from build123d import *

# Parameters (mm, degrees)
BOSS_EXTRUDE1_DEPTH = 6
BOSS_EXTRUDE2_DEPTH = 2.5
BOSS_EXTRUDE4_DEPTH = 2.5
BOSS_EXTRUDE5_DEPTH = 2.5
FILLET1_R           = 2.5
SKETCH6_R           = 2.2
CUT_EXTRUDE1_DEPTH  = 105.505992651
CHAMFER1_SIZE       = 2
SKETCH8_R           = 1.25
BOSS_EXTRUDE6_DEPTH = 2.5
SKETCH10_W          = 2.5
SKETCH10_H          = 5
BOSS_EXTRUDE8_DEPTH = 7.5
SKETCH11_W          = 5
SKETCH11_H          = 2.5
BOSS_EXTRUDE9_DEPTH = 15
FILLET2_R           = 1


with BuildPart() as part:
    # Sketch1 → Boss-Extrude1 (new body)
    with BuildSketch(Plane(origin=(0, 0, 0), x_dir=(1, 0, 0), z_dir=(0, 1, 0))):
        with BuildLine():
            Line((44.658133395, 16.413194813), (15.158133395, 28.913194813))
            ThreePointArc((15.158133395, 28.913194813), (14.345997058, 29.164947656), (13.5, 29.25))
            Line((13.5, 29.25), (-13.5, 29.25))
            ThreePointArc((-13.5, 29.25), (-14.345997058, 29.164947656), (-15.158133395, 28.913194813))
            Line((-15.158133395, 28.913194813), (-44.658133395, 16.413194813))
            ThreePointArc((-44.658133395, 16.413194813), (-46.543272988, 14.846852474), (-47.25, 12.5))
            Line((-47.25, 12.5), (-47.25, -12.5))
            ThreePointArc((-47.25, -12.5), (-46.543272988, -14.846852474), (-44.658133395, -16.413194813))
            Line((-44.658133395, -16.413194813), (-15.158133395, -28.913194813))
            ThreePointArc((-15.158133395, -28.913194813), (-14.345997058, -29.164947656), (-13.5, -29.25))
            Line((-13.5, -29.25), (13.5, -29.25))
            ThreePointArc((13.5, -29.25), (14.345997058, -29.164947656), (15.158133395, -28.913194813))
            Line((15.158133395, -28.913194813), (44.658133395, -16.413194813))
            ThreePointArc((44.658133395, -16.413194813), (46.543272988, -14.846852474), (47.25, -12.5))
            Line((47.25, -12.5), (47.25, 12.5))
            ThreePointArc((47.25, 12.5), (46.543272988, 14.846852474), (44.658133395, 16.413194813))
        make_face()
        with BuildLine():
            Line((43.68276081, 14.111315511), (14.18276081, 26.611315511))
            ThreePointArc((14.18276081, 26.611315511), (13.84835173, 26.714978447), (13.5, 26.75))
            Line((13.5, 26.75), (-13.5, 26.75))
            ThreePointArc((-13.5, 26.75), (-13.84835173, 26.714978447), (-14.18276081, 26.611315511))
            Line((-14.18276081, 26.611315511), (-43.68276081, 14.111315511))
            ThreePointArc((-43.68276081, 14.111315511), (-44.45899476, 13.466351019), (-44.75, 12.5))
            Line((-44.75, 12.5), (-44.75, -12.5))
            ThreePointArc((-44.75, -12.5), (-44.45899476, -13.466351019), (-43.68276081, -14.111315511))
            Line((-43.68276081, -14.111315511), (-14.18276081, -26.611315511))
            ThreePointArc((-14.18276081, -26.611315511), (-13.84835173, -26.714978447), (-13.5, -26.75))
            Line((-13.5, -26.75), (13.5, -26.75))
            ThreePointArc((13.5, -26.75), (13.84835173, -26.714978447), (14.18276081, -26.611315511))
            Line((14.18276081, -26.611315511), (43.68276081, -14.111315511))
            ThreePointArc((43.68276081, -14.111315511), (44.45899476, -13.466351019), (44.75, -12.5))
            Line((44.75, -12.5), (44.75, 12.5))
            ThreePointArc((44.75, 12.5), (44.45899476, 13.466351019), (43.68276081, 14.111315511))
        make_face(mode=Mode.SUBTRACT)
    extrude(amount=BOSS_EXTRUDE1_DEPTH)

    # Sketch2 → Boss-Extrude2 (add)
    with BuildSketch(Plane(origin=(0, 6, 0), x_dir=(1, 0, 0), z_dir=(0, 1, 0))):
        with BuildLine():
            Line((-44.658133395, -16.413194813), (-15.158133395, -28.913194813))
            ThreePointArc((-15.158133395, -28.913194813), (-14.345997058, -29.164947656), (-13.5, -29.25))
            Line((-13.5, -29.25), (13.5, -29.25))
            ThreePointArc((13.5, -29.25), (14.345997058, -29.164947656), (15.158133395, -28.913194813))
            Line((15.158133395, -28.913194813), (44.658133395, -16.413194813))
            ThreePointArc((44.658133395, -16.413194813), (46.543272988, -14.846852474), (47.25, -12.5))
            Line((47.25, -12.5), (47.25, 12.5))
            ThreePointArc((47.25, 12.5), (46.543272988, 14.846852474), (44.658133395, 16.413194813))
            Line((44.658133395, 16.413194813), (15.158133395, 28.913194813))
            ThreePointArc((15.158133395, 28.913194813), (14.345997058, 29.164947656), (13.5, 29.25))
            Line((13.5, 29.25), (-13.5, 29.25))
            ThreePointArc((-13.5, 29.25), (-14.345997058, 29.164947656), (-15.158133395, 28.913194813))
            Line((-15.158133395, 28.913194813), (-44.658133395, 16.413194813))
            ThreePointArc((-44.658133395, 16.413194813), (-46.543272988, 14.846852474), (-47.25, 12.5))
            Line((-47.25, 12.5), (-47.25, -12.5))
            ThreePointArc((-47.25, -12.5), (-46.543272988, -14.846852474), (-44.658133395, -16.413194813))
        make_face()
    extrude(amount=BOSS_EXTRUDE2_DEPTH)

    # Sketch4 → Boss-Extrude4 (add)
    with BuildSketch(Plane(origin=(47.25, 0, 0), x_dir=(0, 0, -1), z_dir=(1, 0, 0))):
        Polygon((-7.5, 0), (7.5, 0), (5, -33.7), (-5, -33.7), align=None)
    extrude(amount=-BOSS_EXTRUDE4_DEPTH)

    # Sketch5 → Boss-Extrude5 (add)
    with BuildSketch(Plane.ZY.offset(47.25)):
        Polygon((7.5, 0), (5, -33.7), (-5, -33.7), (-7.5, 0), align=None)
    extrude(amount=-BOSS_EXTRUDE5_DEPTH)

    # Fillet1
    fillet1_edges = [part.edges().sort_by_distance(p)[0] for p in [
        (46, -33.7, -5),
        (46, 0, -7.5),
        (46, 0, 7.5),
        (46, -33.7, 5),
        (-46, -33.7, -5),
        (-46, -33.7, 5),
        (-46, 0, 7.5),
        (-46, 0, -7.5),
    ]]
    fillet(fillet1_edges, radius=FILLET1_R)

    # Sketch6 → Cut-Extrude1 (cut, through all)
    with BuildSketch(Plane(origin=(47.25, 0, 0), x_dir=(0, 0, -1), z_dir=(1, 0, 0))):
        with Locations((0, -2.3)):
            Circle(SKETCH6_R)
        with Locations((0, -27.7)):
            Circle(SKETCH6_R)
    extrude(amount=-CUT_EXTRUDE1_DEPTH, mode=Mode.SUBTRACT)

    # Chamfer1
    chamfer1_edges = [part.edges().sort_by_distance(p)[0] for p in [
        (-47.25, -2.3, 2.2),
        (47.25, -2.3, 2.2),
        (-47.25, -27.7, 2.2),
        (47.25, -27.7, 2.2),
    ]]
    chamfer(chamfer1_edges, length=CHAMFER1_SIZE)

    # Sketch8 → Boss-Extrude6 (add)
    with BuildSketch(Plane(origin=(0, 6, 0), x_dir=(-1, 0, 0), z_dir=(0, -1, 0))):
        with Locations(Location((40, 10.512979117, 0), (0, 0, 270))):
            Circle(SKETCH8_R)
        with Locations(Location((16.5, 20.470606235, 0), (0, 0, 270))):
            Circle(SKETCH8_R)
        with Locations(Location((-16.5, -20.470606235, 0), (0, 0, 270))):
            Circle(SKETCH8_R)
        with Locations(Location((-40, -10.512979117, 0), (0, 0, 270))):
            Circle(SKETCH8_R)
        with Locations(Location((-40, 10.512979117, 0), (0, 0, 270))):
            Circle(SKETCH8_R)
        with Locations(Location((-16.5, 20.470606235, 0), (0, 0, 270))):
            Circle(SKETCH8_R)
        with Locations(Location((40, -10.512979117, 0), (0, 0, 270))):
            Circle(SKETCH8_R)
        with Locations(Location((16.5, -20.470606235, 0), (0, 0, 270))):
            Circle(SKETCH8_R)
    extrude(amount=BOSS_EXTRUDE6_DEPTH)

    # Sketch10 → Boss-Extrude8 (add)
    with BuildSketch(Plane(origin=(0, 6, 0), x_dir=(-1, 0, 0), z_dir=(0, -1, 0))):
        with Locations((7.5, 0)):
            Rectangle(SKETCH10_W, SKETCH10_H)
    extrude(amount=BOSS_EXTRUDE8_DEPTH)

    # Sketch11 → Boss-Extrude9 (add)
    with BuildSketch(Plane.ZY.offset(6.25)):
        with Locations((0, -0.25)):
            Rectangle(SKETCH11_W, SKETCH11_H)
    extrude(amount=-BOSS_EXTRUDE9_DEPTH)

    # Fillet2
    fillet2_edges = [part.edges().sort_by_distance(p)[0] for p in [
        (-6.25, 6, 0),
        (-7.5, 6, 2.5),
        (-8.75, 6, 0),
        (-7.5, 6, -2.5),
        (-8.75, -1.5, 0),
        (8.75, -1.5, 0),
        (8.75, 1, 0),
        (-6.25, 1, 0),
    ]]
    fillet(fillet2_edges, radius=FILLET2_R)


solid = part.part
Design review of the part built by this model. Coordinates are the model's own, in mm. A direction names the side the tool comes from. Round coordinates to 2 decimals unless told otherwise and drop trailing zeros. Write each loop counter-clockwise with the first axis right and the second up, starting at its lowest first coordinate (ties: lowest second). Pieces come first, ordered by that corner, then holes. Notation, with made-up numbers: (81.25, -21.75) -> (134.25, -21.75) arc R13 ccw to (134.25, -4.75) -> close; hole circle Ø5 at (-22.5, 40.25). An arc over 180 degrees is marked (long way). One line per item, written item: value. Start each with the question number.
Q1. Add section C-C (x = -35.5). Give the boundary of the cut face in (y, z).
Q2. Tool access review of faces 1 (the face through (0, 4, 29.25)), 2 (the face through (0, 0, -2.5)): name each direction out of +Z, -Z, +X, -X, +Y, -Y from which nothing blocks a thin tool from reaching the whole face with its end or side.
Q3. To check wall thickness, follow probe 1 along Y at (x, z) = (-45, 0); probe 2 along X at (y, z) = (-25, 5); probe 3 along Y at (x, z) = (-4.5, 2). State the ranges of each line that lie inside material, in increasing order.
Q4. Add section D-D (x = 16.5). Give the boundary of the cut face in (y, z), then the cut area to 3 significant figures.
Q5. The part is to be moulded in two halves that separate along X. For faces 3 (the face through (28.726, 2.958, 20.449)), 4 (the face through (-17.345, 4.768, -21.392)), 5 (the face through (-47.25, -8, 0)), 6 (the face through (45.98, -0.65, 8.14)), say which applies: pulls with the +X half, pulls with the -X half, needs draft (parallel to the pull), parting line crosses it, or undercut.
Q6. Add section B-B (z = 0). State how many separate pieces and enclosed holes the cut face has, then the cut area to 3 significant figures.
Q7. Add section A-A (x = 2). Give the boundary of the cut face in (y, z), then the cut area to 3 significant figures.
Q8. Insertion check: P1, Ø2, axis at x = 17, z = 20, coming from the -Y side; P2, Ø21.5, axis at x = 6.5, z = 22, coming from the -Y side; P3, Ø6, axis at x = 27.5, z = -11, coming from the -Y side. Each pin has a flat end and moves straight along its axis. Give the tip position at first contact, or say it passes through.
Response:
1. outline: (0, -20.29) -> (8.5, -20.29) -> (8.5, 20.29) -> (0, 20.29) -> (0, 17.58) -> (6, 17.58) -> (6, -17.58) -> (0, -17.58) -> close
2. face 1: +Z, +X, -X, +Y, -Y
2. face 2: -Y
3. probe 1: y = -33.7 to -29.9, -25.5 to -4.5, -0.1 to 8.5
3. probe 2: x = -47.25 to -44.75, 44.75 to 47.25
3. probe 3: y = -1.5 to 1, 6 to 8.5
4. outline: (0, -28.34) -> (8.5, -28.34) -> (8.5, 28.34) -> (0, 28.34) -> (0, 25.63) -> (6, 25.63) -> (6, 21.72) -> (3.5, 21.72) -> (3.5, 19.22) -> (6, 19.22) -> (6, -19.22) -> (3.5, -19.22) -> (3.5, -21.72) -> (6, -21.72) -> (6, -25.63) -> (0, -25.63) -> close
4. area: 187 mm^2
5. face 3: undercut
5. face 4: undercut
5. face 5: pulls with the -X half
5. face 6: needs draft
6. separate pieces: 5
6. enclosed holes: 0
6. area: 431 mm^2
7. outline: (-1.5, -2.5) -> (1, -2.5) -> (1, 2.5) -> (-1.5, 2.5) -> close; (0, -29.25) -> (8.5, -29.25) -> (8.5, 29.25) -> (0, 29.25) -> (0, 26.75) -> (6, 26.75) -> (6, -26.75) -> (0, -26.75) -> close
7. area: 189 mm^2
8. P1: stops at y = 3.5
8. P2: stops at y = 0
8. P3: stops at y = 6
